Geometry check sheet. Reference: the model listing, model coordinates, mm. Round coordinates to 2 decimals unless told otherwise and drop trailing zeros. Write each loop counter-clockwise with the first axis right and the second up, starting at its lowest first coordinate (ties: lowest second). Pieces come first, ordered by that corner, then holes. Notation, with made-up numbers: M 64.5,-18.75 L 117.5,-18.75 A23 ccw 117.5,-4.75 Z; hole C 8.5,-37.5 d2. An arc over 180 degrees is marked long. Answer in a Markdown table with one row per item. Add a question column.
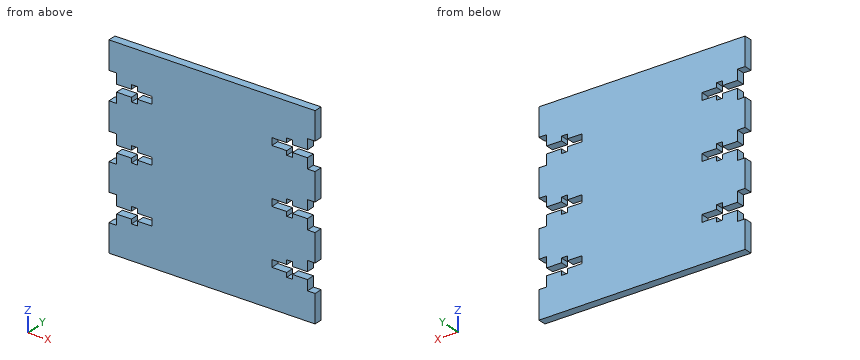
from build123d import *

# Parameters (mm, degrees)
SKETCH1_W                 = 75
SKETCH1_H                 = 77
BOSS_EXTRUDE1_DEPTH       = 3.2
SKETCH2_W                 = 3
SKETCH2_H                 = 11
BOSS_EXTRUDE3_DEPTH       = 3.2
LPATTERN1_COUNT           = 4
LPATTERN1_PITCH           = 22
SKETCH4_W                 = 3
SKETCH4_H                 = 11
BOSS_EXTRUDE5_DEPTH       = 3.2
LPATTERN2_COUNT           = 4
LPATTERN2_PITCH           = 22
SKETCH5_W                 = 14
SKETCH5_H                 = 2.85
SKETCH5_W_2               = 2.3
SKETCH5_H_2               = 6.3
CUT_EXTRUDE1_DEPTH        = 56.970885289
LPATTERN3_COUNT           = 3
LPATTERN3_PITCH           = 22
MIRROR1_COPY_1_SKETCH_W   = 14
MIRROR1_COPY_1_SKETCH_H   = 2.85
MIRROR1_COPY_1_SKETCH_W_2 = 2.3
MIRROR1_COPY_1_SKETCH_H_2 = 6.3
MIRROR1_COPY_1_DEPTH      = 56.970885289
MIRROR1_COPY_2_SKETCH_W   = 14
MIRROR1_COPY_2_SKETCH_H   = 2.85
MIRROR1_COPY_2_SKETCH_W_2 = 2.3
MIRROR1_COPY_2_SKETCH_H_2 = 6.3
MIRROR1_COPY_2_DEPTH      = 56.970885289


with BuildPart() as part:
    # Sketch1 → Boss-Extrude1 (new body)
    with BuildSketch(Plane(origin=(0, 0, 0), x_dir=(1, 0, 0), z_dir=(0, 1, 0))):
        Rectangle(SKETCH1_W, SKETCH1_H)
    extrude(amount=BOSS_EXTRUDE1_DEPTH)

    # Sketch2 → Boss-Extrude3 (add)
    with BuildSketch(Plane(origin=(0, 3.2, 0), x_dir=(1, 0, 0), z_dir=(0, 1, 0))):
        with Locations((-39, 33)):
            Rectangle(SKETCH2_W, SKETCH2_H)
    boss_extrude3 = extrude(amount=-BOSS_EXTRUDE3_DEPTH)

    # LPattern1: Boss-Extrude3 ×4
    with Locations(*[(0, 0, i * LPATTERN1_PITCH) for i in range(1, LPATTERN1_COUNT)]):
        add(boss_extrude3)

    # Sketch4 → Boss-Extrude5 (add)
    with BuildSketch(Plane(origin=(0, 3.2, 0), x_dir=(1, 0, 0), z_dir=(0, 1, 0))):
        with Locations((39, 33)):
            Rectangle(SKETCH4_W, SKETCH4_H)
    boss_extrude5 = extrude(amount=-BOSS_EXTRUDE5_DEPTH)

    # LPattern2: Boss-Extrude5 ×4
    with Locations(*[(0, 0, i * LPATTERN2_PITCH) for i in range(1, LPATTERN2_COUNT)]):
        add(boss_extrude5)

    # Sketch5 → Cut-Extrude1 (cut, through all)
    with BuildSketch(Plane(origin=(0, 3.2, 0), x_dir=(1, 0, 0), z_dir=(0, 1, 0))):
        with Locations((-30.5, 22)):
            Rectangle(SKETCH5_W, SKETCH5_H)
        with Locations((-30.5, 22)):
            Rectangle(SKETCH5_W_2, SKETCH5_H_2)
    cut_extrude1 = extrude(amount=-CUT_EXTRUDE1_DEPTH, mode=Mode.SUBTRACT)

    # LPattern3: Cut-Extrude1 ×3
    with Locations(*[(0, 0, i * LPATTERN3_PITCH) for i in range(1, LPATTERN3_COUNT)]):
        add(cut_extrude1, mode=Mode.SUBTRACT)

    # Mirror1: Cut-Extrude1 across plane
    add(cut_extrude1.mirror(Plane(origin=(0, 0, 0), x_dir=(0, 0, 1), z_dir=(1, 0, 0))), mode=Mode.SUBTRACT)

    # Mirror1 copy 1 sketch → Mirror1 copy 1 (cut, through all)
    with BuildSketch(Plane(origin=(0, 3.2, 22), x_dir=(-1, 0, 0), z_dir=(0, 1, 0))):
        with Locations((-30.5, -22)):
            Rectangle(MIRROR1_COPY_1_SKETCH_W, MIRROR1_COPY_1_SKETCH_H)
        with Locations((-30.5, -22)):
            Rectangle(MIRROR1_COPY_1_SKETCH_W_2, MIRROR1_COPY_1_SKETCH_H_2)
    extrude(amount=-MIRROR1_COPY_1_DEPTH, mode=Mode.SUBTRACT)

    # Mirror1 copy 2 sketch → Mirror1 copy 2 (cut, through all)
    with BuildSketch(Plane(origin=(0, 3.2, 44), x_dir=(-1, 0, 0), z_dir=(0, 1, 0))):
        with Locations((-30.5, -22)):
            Rectangle(MIRROR1_COPY_2_SKETCH_W, MIRROR1_COPY_2_SKETCH_H)
        with Locations((-30.5, -22)):
            Rectangle(MIRROR1_COPY_2_SKETCH_W_2, MIRROR1_COPY_2_SKETCH_H_2)
    extrude(amount=-MIRROR1_COPY_2_DEPTH, mode=Mode.SUBTRACT)


solid = part.part
Item 1: Gauge pin test, flat ends, axial feed: pin 1 Ø0.9 at (y, z) = (2, 20) entering from +X; pin 2 Ø1.6 at (y, z) = (1.5, 4) entering from -X. Record the tip position at first contact, or that the pin passes through.
Item 2: Section check B-B, the plane z = -17.5. Record the boundary of the cut face in (x, y).
Item 3: Section check A-A, the plane x = -35.5. Record the boundary of the cut face in (y, z) (3 decimals).
Item 4: Scan lines: probe 1 along X at (y, z) = (0.3, -19.5); probe 2 along X at (y, z) = (2.55, 18); probe 3 along X at (y, z) = (1.2, 21). Record each from-to range of solid material in increasing order. Write a range as from..to.
Result sheet:
| question | item | result |
|---|---|---|
| 1 | pin 1 | stops at x = 37.5 |
| 1 | pin 2 | stops at x = -37.5 |
| 2 | outline | M -37.5,0 L 37.5,0 L 37.5,3.2 L -37.5,3.2 Z |
| 3 | outline | M 0,-38.5 L 3.2,-38.5 L 3.2,-23.425 L 0,-23.425 Z; M 0,-20.575 L 3.2,-20.575 L 3.2,-1.425 L 0,-1.425 Z; M 0,1.425 L 3.2,1.425 L 3.2,20.575 L 0,20.575 Z; M 0,23.425 L 3.2,23.425 L 3.2,38.5 L 0,38.5 Z |
| 4 | probe 1 | x = -37.5..-31.65, -29.35..29.35, 31.65..37.5 |
| 4 | probe 2 | x = -37.5..37.5 |
| 4 | probe 3 | x = -23.5..23.5 |
